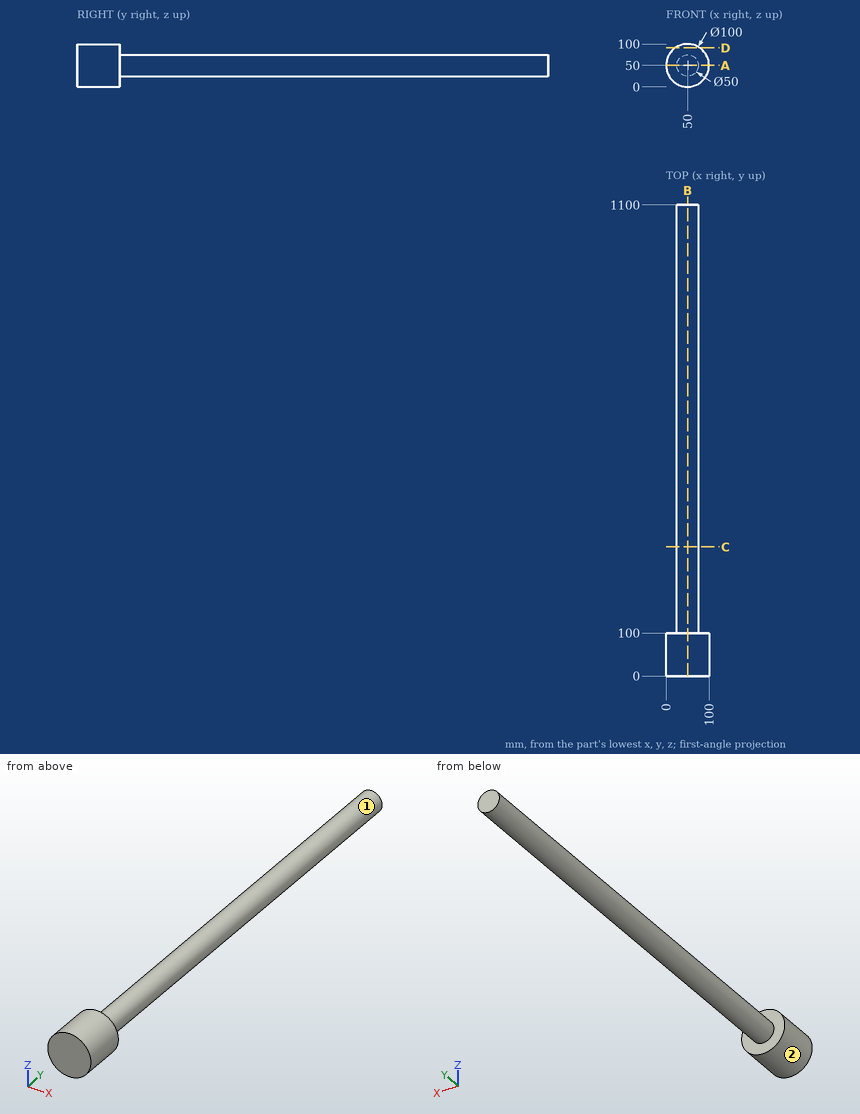
Drawing for the job (mm, zero at the part's lowest x, y, z). A direction names the side the tool comes from. Round coordinates to 2 decimals unless told otherwise and drop trailing zeros. Loops run counter-clockwise (first coordinate to the right, second up) from the corner with the lowest first, then second, coordinate; pieces in that order, holes last. Notation, with made-up numbers: (81.5, -11) - (115.5, -11) arc R27 ccw to (115.5, 5) - close; hole circle Ø7 at (25, -27). An arc over 180 degrees is marked (long way). Return JSON: item names as keys, results as strings. Group by question number.
Q1. Flat gauge pins, fed straight in: pin 1 Ø1 at (x, z) = (79, 31.5) entering from +Y; pin 2 Ø6 at (x, y) = (49.5, 758) entering from -Z; pin 3 Ø1.5 at (x, y) = (41.5, 281) entering from -Z. Where does each tip first touch, or does it go through?
Q2. Tool access for the marked faces 1 and 2: list every direction of +Z, -Z, +X, -X, +Y, -Y with a clear straight run to the whole face (end or side of a thin tool).
Q3. Band-saw the part on A-A on z = 50. Give the cut face in (x, y), plus the area to 3 significant figures.
Q4. Band-saw the part on D-D on z = 91. Give the cut face in (x, y).
Q5. Band-saw the part on C-C on y = 301.5. Give the cut face in (x, z).
Q6. Drill centre lines: line 1 along Y through (x, z) = (83.5, 77.5); line 2 along Z through (x, y) = (50.5, 395) (3 decimals); line 3 along Z through (x, y) = (84, 70.5). Where is each one in solid material? Low to high. Write a range as [from, to].
Q7. Band-saw the part on B-B on x = 50. Give the cut face in (y, z), plus the area to 3 significant figures.
Solutions:
{
 "1": {"pin 1": "stops at y = 100", "pin 2": "stops at z = 25", "pin 3": "stops at z = 26.23"},
 "2": {"face 1": "+Y", "face 2": "+Y, -Y"},
 "3": {"outline": "(0, 0) - (100, 0) - (100, 100) - (75, 100) - (75, 1100) - (25, 1100) - (25, 100) - (0, 100) - close", "area": "60,000 mm^2"},
 "4": {"outline": "(21.38, 0) - (78.62, 0) - (78.62, 100) - (21.38, 100) - close"},
 "5": {"outline": "circle Ø50 at (50, 50)"},
 "6": {"line 1": "y = [0, 100]", "line 2": "z = [25.005, 74.995]", "line 3": "z = [13.34, 86.66]"},
 "7": {"outline": "(0, 0) - (100, 0) - (100, 25) - (1100, 25) - (1100, 75) - (100, 75) - (100, 100) - (0, 100) - close", "area": "60,000 mm^2"}
}
